Autodesk Inventor part; units mm, degrees
ref_plane "YZ Plane" through (0, 0, 0) normal (1, 0, 0) x (0, 1, 0)
ref_plane "XZ Plane" through (0, 0, 0) normal (0, 1, 0) x (-1, 0, 0)
ref_plane "XY Plane" through (0, 0, 0) normal (0, 0, 1) x (1, 0, 0)
sketch "Sketch_1" plane through (0, 0, 0) normal (0, 0, 1) x (1, 0, 0)
  line L0 (25, 0) -> (-15, 0)
  line L1 (-15, 0) -> (-15, 4.5)
  line L2 (-15, 4.5) -> (-14.5, 5)
  line L3 (-14.5, 5) -> (-0.2, 5)
  arc A0 (-0.2, 5) -> (0, 5.2) centre (-0.2, 5.2) ccw
  line L4 (0, 5.2) -> (0, 7)
  line L5 (0, 7) -> (0.5, 7.5)
  line L6 (0.5, 7.5) -> (24.5, 7.5)
  line L7 (24.5, 7.5) -> (25, 7)
  line L8 (25, 7) -> (25, 0)
  line L9 (25, 0) -> (-15, 0)
revolve "Revolution1" add sketch "Sketch_1" angle 360 about axis through (25, 0, 0) along (1, 0, 0)
sketch "Sketch_40" plane through (0, 0, 0) normal (0, 0, 1) x (1, 0, 0)
  line L0 (1000, 0) -> (-1000, 0)
  line L1 (-11.15, 4.8) -> (-10, 4.8)
  line L2 (-10, 4.8) -> (-10, 20)
  line L3 (-10, 20) -> (-11.15, 20)
  line L4 (-11.15, 20) -> (-11.15, 4.8)
revolve "Revolution2" cut sketch "Sketch_40" angle 360 about axis through (1000, 0, 0) along (1, 0, 0)
properties part number "SFRX15-25-F15-B5-P10"
Read the model definition and answer for the solid it produces. Units are mm, in the model's axes. A direction names the side the tool comes from. Give positions to 0.01 mm unless a question says otherwise; leave off trailing zeros. Order: outer loops, then holes, each group sorted by start corner. A loop starts at its lowest first (then second) coordinate and runs counter-clockwise, first axis right, second up. Notation, with made-up numbers: (67.25, 4.5) -> (100.25, 4.5) arc R15 cw to (100.25, 24.5) -> close; hole circle Ø7 at (65, 8.25). An arc over 180 degrees is marked (long way). Write item = value, one per line.
1. A cutting plane is placed at A-A, the plane y = 0. Write down the section's boundary in (x, z).
Numbers:
outline = (-15, -4.5) -> (-14.5, -5) -> (-11.15, -5) -> (-11.15, -4.8) -> (-10, -4.8) -> (-10, -5) -> (-0.2, -5) arc R0.2 cw to (0, -5.2) -> (0, -7) -> (0.5, -7.5) -> (24.5, -7.5) -> (25, -7) -> (25, 7) -> (24.5, 7.5) -> (0.5, 7.5) -> (0, 7) -> (0, 5.2) arc R0.2 cw to (-0.2, 5) -> (-10, 5) -> (-10, 4.8) -> (-11.15, 4.8) -> (-11.15, 5) -> (-14.5, 5) -> (-15, 4.5) -> close
2. Straight lines are drawn through the part: line 1 along X through (y, z) = (4.25, -1.5); line 2 along X through (y, z) = (5.25, -2.5); line 3 along Z through (x, y) = (1, -6). For each, find the intervals that lie inside material, in ascending order.
Numbers:
line_1 = -14.99 to 25
line_2 = 0 to 25
line_3 = -4.5 to 4.5
3. For faces 4 (the face through (-5.03, -1.08, -4.88)), 5 (the face through (-15, 0, 0)), determine the directions among +Z, -Z, +X, -X, +Y, -Y from which every point of the face is accessible in a straight line to the end or side of a thin tool.
Numbers:
face_4 = -X
face_5 = +Z, -Z, -X, +Y, -Y
4. Given pin 1 (6 mm diameter, centred on x = -11, z = 2.5, fed in from +Y); pin 2 (1.5 mm diameter, centred on x = -2.5, y = 4, fed in from +Z); pin 3 (1.5 mm diameter, centred on x = -3, z = 6, fed in from +Y), each flat-ended and moving along its own axis, determine where each tip first touches the part or whether it passes through.
Numbers:
pin_1 = 5
pin_2 = 3.8
pin_3 = through
5. The mould has two halves that part along X. Classify faces 1 (the face through (25, 0, 0)), 2 (the face through (12.668, -7.493, 0.33)), 3 (the face through (-10.57, 2.58, 4.05)): +X half, -X half, draft (parallel to the pull), parting line (faces both ways), or undercut.
Numbers:
face_1 = +X half
face_2 = draft
face_3 = undercut
6. A cutting plane is placed at C-C, the plane x = 10.5. Write down the section's boundary in (y, z), and give its area (3 significant figures).
Numbers:
outline = circle Ø15 at (0, 0)
area = 177 mm²
7. A cutting plane is placed at D-D, the plane x = -9. Write down the section's boundary in (y, z).
Numbers:
outline = circle Ø10 at (0, 0)
